The listing builds one solid part. Answer for the finished solid, in the listing's coordinates (mm). Coordinates: 2 decimals unless noted, no trailing zeros. Write each question's results on one line, items separated by ' | '. Start each with the question number.
(1) A straight line is drawn through the part: L1, parallel to X at y = -69, z = 0.1. Find the intervals that lie inside material, in ascending order.
(2) Given pin 1 (1 mm diameter, centred on x = 111.5, z = 1, fed in from -Y); pin 2 (1 mm diameter, centred on x = 111, z = 0.5, fed in from +Y); pin 3 (1 mm diameter, centred on y = 59, z = 1, fed in from -X), each flat-ended and moving along its own axis, determine where each tip first touches the part or whether it passes through.
(3) Determine the mould class of faces 1 (the face through (-27, -40, 2)), 2 (the face through (-27, -40, 0)) for opening direction Z: +Z half, -Z half, draft (parallel to the pull), parting line (faces both ways), or undercut.
```python
from build123d import *

# Parameters (mm, degrees)
SKETCH1_W               = 274
SKETCH1_H               = 300
BOSS_EXTRUDE1_DEPTH     = 2
SKETCH2_W               = 2
SKETCH2_H               = 20
CUT_EXTRUDE1_DEPTH      = 4
LPATTERN1_COUNT         = 8
LPATTERN1_PITCH         = 40
MIRROR1_COPY_1_SKETCH_W = 2
MIRROR1_COPY_1_SKETCH_H = 20
MIRROR1_COPY_1_DEPTH    = 4
MIRROR1_COPY_2_SKETCH_W = 2
MIRROR1_COPY_2_SKETCH_H = 20
MIRROR1_COPY_2_DEPTH    = 4
MIRROR1_COPY_3_SKETCH_W = 2
MIRROR1_COPY_3_SKETCH_H = 20
MIRROR1_COPY_3_DEPTH    = 4
MIRROR1_COPY_4_SKETCH_W = 2
MIRROR1_COPY_4_SKETCH_H = 20
MIRROR1_COPY_4_DEPTH    = 4
MIRROR1_COPY_5_SKETCH_W = 2
MIRROR1_COPY_5_SKETCH_H = 20
MIRROR1_COPY_5_DEPTH    = 4
MIRROR1_COPY_6_SKETCH_W = 2
MIRROR1_COPY_6_SKETCH_H = 20
MIRROR1_COPY_6_DEPTH    = 4
MIRROR1_COPY_7_SKETCH_W = 2
MIRROR1_COPY_7_SKETCH_H = 20
MIRROR1_COPY_7_DEPTH    = 4


with BuildPart() as part:
    # Sketch1 → Boss-Extrude1 (new body)
    with BuildSketch(Plane.XY):
        with Locations((-24.689291101, -42.156862745)):
            Rectangle(SKETCH1_W, SKETCH1_H)
    extrude(amount=BOSS_EXTRUDE1_DEPTH)

    # Sketch2 → Cut-Extrude1 (cut)
    with BuildSketch(Plane.XY.offset(2)):
        with Locations((-160.689291101, 97.843137255)):
            Rectangle(SKETCH2_W, SKETCH2_H)
    cut_extrude1 = extrude(amount=-CUT_EXTRUDE1_DEPTH, mode=Mode.SUBTRACT)

    # LPattern1: Cut-Extrude1 ×8
    with Locations(*[(0, -i * LPATTERN1_PITCH, 0) for i in range(1, LPATTERN1_COUNT)]):
        add(cut_extrude1, mode=Mode.SUBTRACT)

    # Mirror1: Cut-Extrude1 across plane
    add(cut_extrude1.mirror(Plane.ZY.offset(24.689291101)), mode=Mode.SUBTRACT)

    # Mirror1 copy 1 sketch → Mirror1 copy 1 (cut)
    with BuildSketch(Plane(origin=(-49.378582202, -40, 2), x_dir=(-1, 0, 0), z_dir=(0, 0, 1))):
        with Locations((-160.689291101, -97.843137255)):
            Rectangle(MIRROR1_COPY_1_SKETCH_W, MIRROR1_COPY_1_SKETCH_H)
    extrude(amount=-MIRROR1_COPY_1_DEPTH, mode=Mode.SUBTRACT)

    # Mirror1 copy 2 sketch → Mirror1 copy 2 (cut)
    with BuildSketch(Plane(origin=(-49.378582202, -80, 2), x_dir=(-1, 0, 0), z_dir=(0, 0, 1))):
        with Locations((-160.689291101, -97.843137255)):
            Rectangle(MIRROR1_COPY_2_SKETCH_W, MIRROR1_COPY_2_SKETCH_H)
    extrude(amount=-MIRROR1_COPY_2_DEPTH, mode=Mode.SUBTRACT)

    # Mirror1 copy 3 sketch → Mirror1 copy 3 (cut)
    with BuildSketch(Plane(origin=(-49.378582202, -120, 2), x_dir=(-1, 0, 0), z_dir=(0, 0, 1))):
        with Locations((-160.689291101, -97.843137255)):
            Rectangle(MIRROR1_COPY_3_SKETCH_W, MIRROR1_COPY_3_SKETCH_H)
    extrude(amount=-MIRROR1_COPY_3_DEPTH, mode=Mode.SUBTRACT)

    # Mirror1 copy 4 sketch → Mirror1 copy 4 (cut)
    with BuildSketch(Plane(origin=(-49.378582202, -160, 2), x_dir=(-1, 0, 0), z_dir=(0, 0, 1))):
        with Locations((-160.689291101, -97.843137255)):
            Rectangle(MIRROR1_COPY_4_SKETCH_W, MIRROR1_COPY_4_SKETCH_H)
    extrude(amount=-MIRROR1_COPY_4_DEPTH, mode=Mode.SUBTRACT)

    # Mirror1 copy 5 sketch → Mirror1 copy 5 (cut)
    with BuildSketch(Plane(origin=(-49.378582202, -200, 2), x_dir=(-1, 0, 0), z_dir=(0, 0, 1))):
        with Locations((-160.689291101, -97.843137255)):
            Rectangle(MIRROR1_COPY_5_SKETCH_W, MIRROR1_COPY_5_SKETCH_H)
    extrude(amount=-MIRROR1_COPY_5_DEPTH, mode=Mode.SUBTRACT)

    # Mirror1 copy 6 sketch → Mirror1 copy 6 (cut)
    with BuildSketch(Plane(origin=(-49.378582202, -240, 2), x_dir=(-1, 0, 0), z_dir=(0, 0, 1))):
        with Locations((-160.689291101, -97.843137255)):
            Rectangle(MIRROR1_COPY_6_SKETCH_W, MIRROR1_COPY_6_SKETCH_H)
    extrude(amount=-MIRROR1_COPY_6_DEPTH, mode=Mode.SUBTRACT)

    # Mirror1 copy 7 sketch → Mirror1 copy 7 (cut)
    with BuildSketch(Plane(origin=(-49.378582202, -280, 2), x_dir=(-1, 0, 0), z_dir=(0, 0, 1))):
        with Locations((-160.689291101, -97.843137255)):
            Rectangle(MIRROR1_COPY_7_SKETCH_W, MIRROR1_COPY_7_SKETCH_H)
    extrude(amount=-MIRROR1_COPY_7_DEPTH, mode=Mode.SUBTRACT)


solid = part.part
```
Established:
1) L1: x = -159.69 to 110.31
2) pin 1: stops at y = -172.16 | pin 2: stops at y = 87.84 | pin 3: stops at x = -159.69
3) face 1: +Z half | face 2: -Z half
